Check sheet for the modelled part. Datum: model origin and axes. Units: mm. A direction names the side the tool comes from. Coordinates: 2 decimals unless noted, no trailing zeros. Write each loop counter-clockwise with the first axis right and the second up, starting at its lowest first coordinate (ties: lowest second). Pieces come first, ordered by that corner, then holes. Notation, with made-up numbers: (31, -19) -> (83, -19) arc R25 cw to (83, 5) -> close; hole circle Ø6 at (9, -40). An arc over 180 degrees is marked (long way). Put each result on its own line as item: value.
Autodesk Inventor part; units mm, degrees
ref_plane "YZ Plane" through (0, 0, 0) normal (1, 0, 0) x (0, 1, 0)
ref_plane "XZ Plane" through (0, 0, 0) normal (0, 1, 0) x (-1, 0, 0)
ref_plane "XY Plane" through (0, 0, 0) normal (0, 0, 1) x (1, 0, 0)
sketch "スケッチ1" plane through (0, 0, 0) normal (0, 1, 0) x (-1, 0, 0)
  line L0 (0, 0) -> (115, 0)
  line L1 (115, 0) -> (115, -157)
  line L2 (115, -157) -> (0, -157)
  line L3 (0, -157) -> (0, 0)
  line L4 (120, -162) -> (120, 5)
  line L5 (120, 5) -> (-5, 5)
  line L6 (-5, 5) -> (-5, -162)
  line L7 (-5, -162) -> (120, -162)
  dimension "d0" = 115
  dimension "d1" = 157
  dimension "d2" = 5
extrude "押し出し1" add sketch "スケッチ1" along normal blind 5 contours L0 L1 L2 L3 | L7 L6 L5 L4
sketch "スケッチ2" plane through (0, 5, 0) normal (0, 1, 0) x (1, 0, 0)
  line L0 (-120, -5) -> (5, -5)
  line L1 (5, -5) -> (5, 162)
  line L2 (5, 162) -> (-120, 162)
  line L3 (-120, 162) -> (-120, -5)
  line L4 (-115, 0) -> (0, 0)
  line L5 (0, 0) -> (0, 157)
  line L6 (0, 157) -> (-115, 157)
  line L7 (-115, 157) -> (-115, 0)
  line L8 (-115, 0) -> (-120, 0)
  line L9 (-120, 162) -> (-120, -5)
  line L10 (-115, 157) -> (-120, 157)
  point P0 (0, 0)
  dimension "d5" = 5
extrude "押し出し2" add sketch "スケッチ2" along normal blind 20 contours L3 L8 L4 L5 L6 L10 L2 L1 L0
sketch "スケッチ3" plane through (0, 5, -157) normal (-1, 0, 0) x (0, 0, 1)
  line L0 (0, 0) -> (0, 20)
  line L1 (0, 20) -> (3, 20)
  line L2 (0, 20) -> (157, 20)
  line L3 (3, 20) -> (3, 18.5)
  line L4 (3, 18.5) -> (0, 17)
  line L5 (78.5, 20) -> (78.5, -5)
  line L6 (-5, -5) -> (162, -5)
  line L7 (157, 20) -> (154, 20)
  line L8 (154, 20) -> (154, 18.5)
  line L9 (154, 18.5) -> (157, 17)
  line L10 (157, 0) -> (0, 0)
  line L11 (157, 0) -> (157, 20)
  line L12 (0, 20) -> (157, 20)
  line L13 (0, 0) -> (0, 20)
  point P0 (157, -5)
  point P1 (157, 17)
  point P2 (154, 20)
  dimension "d8" = 3
  dimension "d9" = 1.5
  dimension "d10" = 1.5
extrude "押し出し3" add sketch "スケッチ3" along normal blind 85 contours L0 L1 L3 L4 | L2 L11 L9 L8
sketch "スケッチ4" plane through (-120, 0, 5) normal (0, 0, 1) x (1, 0, 0)
  line L0 (120, 25) -> (35, 25)
  line L1 (65, 25) -> (25, 25)
  line L2 (25, 25) -> (25, 5)
  line L3 (25, 5) -> (65, 5)
  line L4 (65, 5) -> (65, 25)
  line L5 (0, 0) -> (0, 25)
  line L6 (0, 5) -> (120, 5)
  line L7 (25, 23) -> (65, 23)
  point P0 (120, 0)
  dimension "d13" = 65
  dimension "d14" = 40
  dimension "d15" = 0
  dimension "d16" = 2
extrude "押し出し4" cut sketch "スケッチ4" against normal blind 10 contours L4 L3 L2 L7
sketch "スケッチ5" plane through (0, 0, 0) normal (0, -1, 0) x (1, 0, 0)
  line L0 (-95, -116) -> (-55, -116)
  line L1 (-55, -116) -> (-55, -41)
  line L2 (-55, -41) -> (-95, -41)
  line L3 (-95, -41) -> (-95, -116)
  line L4 (-120, -162) -> (-120, 5)
  point P0 (0, 0)
  point P1 (-120, -78.5)
  point P2 (-95, -78.5)
  dimension "d19" = 65
  dimension "d20" = 75
  dimension "d21" = 25
  dimension "d22" = 0
extrude "押し出し5" cut sketch "スケッチ5" against normal through all
sketch "スケッチ6" plane through (5, 0, 5) normal (1, 0, 0) x (0, 0, -1)
  line L0 (5, 5) -> (5, 22)
  line L1 (5, 5) -> (30, 5)
  line L2 (30, 5) -> (30, 22)
  line L3 (30, 22) -> (5, 22)
  line L4 (5, 22) -> (5, 5)
  point P0 (5, 0)
  dimension "d25" = 25
  dimension "d26" = 0
extrude "押し出し6" cut sketch "スケッチ6" against normal up to surface (5 mm away)
sketch "スケッチ7" plane through (0, 0, 0) normal (0, -1, 0) x (1, 0, 0)
  circle A0 centre (-115, 15) radius 1.7
  circle A1 centre (0, 15) radius 1.7
  circle A2 centre (-115, -172) radius 1.7
  circle A3 centre (0, -172) radius 1.7
  line L0 (5, -162) -> (-120, -162)
  line L1 (-5, -162) -> (5, -162)
  line L2 (5, -162) -> (5, -177)
  line L3 (5, -177) -> (-5, -177)
  line L4 (-5, -177) -> (-5, -162)
  line L5 (-110, -162) -> (-120, -162)
  line L6 (-120, -162) -> (-120, -177)
  line L7 (-120, -177) -> (-110, -177)
  line L8 (-110, -177) -> (-110, -162)
  line L9 (-120, 5) -> (5, 5)
  line L10 (-120, 5) -> (-110, 5)
  line L11 (-110, 5) -> (-110, 20)
  line L12 (-110, 20) -> (-120, 20)
  line L13 (-120, 20) -> (-120, 5)
  line L14 (-5, 5) -> (5, 5)
  line L15 (5, 5) -> (5, 20)
  line L16 (5, 20) -> (-5, 20)
  line L17 (-5, 20) -> (-5, 5)
  line L18 (5, 5) -> (5, -162)
  line L19 (-120, -162) -> (-120, 5)
  circle A4 centre (120, -172) radius 1.7
  circle A5 centre (62.9804, -172) radius 1.525
  point P0 (0, 0)
  dimension "d29" = 3.4
  dimension "d30" = 3.4
  dimension "d31" = 3.4
  dimension "d32" = 3.4
  dimension "d33" = 5
  dimension "d34" = 5
  dimension "d35" = 5
  dimension "d36" = 5
  dimension "d37" = 5
  dimension "d38" = 5
  dimension "d39" = 5
  dimension "d40" = 5
  dimension "d41" = 5
  dimension "d42" = 5
  dimension "d43" = 5
  dimension "d44" = 5
  dimension "d45" = 10
  dimension "d46" = 10
  dimension "d47" = 10
  dimension "d48" = 10
  dimension "d56" = 0
  dimension "d57" = 0
  dimension "d60" = 57.0196
  dimension "d63" = 0
  dimension "d64" = 0
extrude "押し出し7" add sketch "スケッチ7" against normal blind 5 contours L2 L3 L4 L0 | L9 L17 L16 L15 | L8 L7 L6 L0 | L9 L13 L12 L11
fillet "フィレット1" radius 2 8 edges at (-110, 2.5, 5) (-5, 2.5, 5) (-110, 2.5, -162) (-5, 2.5, -162) (0, 5, -162) (-115, 5, -162) (-115, 5, 5) (0, 5, 5)
fillet "フィレット2" radius 1 37 edges at (5, 5, 13.5) (5, 16, 5) (5, 2.5, 20) (-57.5, 25, 5) (-110, 2.5, 20) (-120, 2.5, 20) (-5, 2.5, -177) (-57.5, 25, -162) (5, 25, -78.5) (5, 5, -170.5) (5, 16, -162) (-5.5858, 5.5858, -162.5858) (-5, 5, -170.5) (0, 5, -177) (-115, 5, -177) (-109.4142, 5.5858, -162.5858) (-110, 5, -170.5) (-120, 2.5, -177) (-110, 2.5, -177) (-120, 16, -162) (-120, 5, -170.5) (-120, 5, 13.5) (-120, 16, 5) (-109.4142, 5.5858, 5.5858) (-110, 5, 13.5) (-115, 5, 20) (-42.5, 25, -3) (-102.5, 25, 0) (0, 25, -78.5) (-42.5, 25, -154) (-102.5, 25, -157) (-85, 25, -155.5) (-85, 25, -1.5) (-95, 2.5, -41) (-55, 2.5, -41) (-55, 2.5, -116) (-95, 2.5, -116)
properties part number "pccase"
Q1. Depth check by flat-ended pin: P1, Ø3, axis at x = -87.5, z = -141, coming from the -Y side; P2, Ø6.5, axis at x = -2, z = -171, coming from the +Y side; P3, Ø0.6, axis at x = -23, y = 24, coming from the +Z side; P4, Ø4, axis at x = -72.5, y = 19.5, coming from the +Z side. Enter the tip coordinate at first touch or a pass-through.
Recorded:
P1: stops at y = 0
P2: stops at y = 5
P3: stops at z = 5
P4: stops at z = -157
Q2. Material ranges on line 1 along Z through (x, y) = (-115, 3.8); line 2 along Z through (x, y) = (-58, 4.5); line 3 along X through (y, z) = (1.5, -172), recorded low to high.
Recorded:
line 1: z = -177 to -173.7, -170.3 to 13.3, 16.7 to 20
line 2: z = -162 to -116, -41 to 5
line 3: x = -120 to -116.7, -113.3 to -110, -5 to -1.7, 1.7 to 5
Q3. Cross-section at A-A (x = -88.5). Record the cut outline in (y, z), plus the area to 3 significant figures.
Recorded:
outline: (0, -162) -> (24, -162) arc R1 ccw to (25, -161) -> (25, -158) arc R1 ccw to (24, -157) -> (5, -157) -> (5, -116) -> (0, -116) -> close; (0, -41) -> (5, -41) -> (5, 5) -> (0, 5) -> close; (23, 0) -> (24, 0) arc R1 ccw to (25, 1) -> (25, 4) arc R1 ccw to (24, 5) -> (23, 5) -> close
area: 569 mm2
Q4. Tool access check on faces 4 (the flat face through (-75, 2, -116)), 5 (the flat face through (-5, 2, 14)), 6 (the flat face through (-5, 2, -170)), 7 (the flat face through (-59, 14, -157)). Record the directions out of +Z, -Z, +X, -X, +Y, -Y that give a thin tool (end or side, any length) a straight path to the whole face; none if there is none.
Recorded:
face 4: +Y, -Y
face 5: +Z, +Y, -Y
face 6: -Z, +Y, -Y
face 7: -X
Q5. Cross-section at C-C (y = 19.5). Record the cut outline in (x, z).
Recorded:
outline: (-120, -161) arc R1 ccw to (-119, -162) -> (4, -162) arc R1 ccw to (5, -161) -> (5, -25) -> (0, -25) -> (0, -157) -> (-120, -157) -> close; (-120, 0) -> (-95, 0) -> (-95, 5) -> (-119, 5) arc R1 ccw to (-120, 4) -> close; (-55, 0) -> (5, 0) -> (5, 4) arc R1 ccw to (4, 5) -> (-55, 5) -> close
Q6. Mould release check, pull along Z, two halves, no side actions. Record for faces 1 (the flat face through (1, 2, -177)), 2 (the flat face through (-95, 2, -78)), 3 (the flat face through (-45, 12, 5)): released by +Z, released by -Z, zero draft, split by the parting line, or undercut.
Recorded:
face 1: released by -Z
face 2: undercut
face 3: released by +Z
Q7. Cross-section at D-D (x = -19). Record the cut outline in (y, z), plus the area to 3 significant figures.
Recorded:
outline: (0, -162) -> (24, -162) arc R1 ccw to (25, -161) -> (25, -155) arc R1 ccw to (24, -154) -> (23.5, -154) -> (22, -157) -> (5, -157) -> (5, 0) -> (22, 0) -> (23.5, -3) -> (24, -3) arc R1 ccw to (25, -2) -> (25, 4) arc R1 ccw to (24, 5) -> (0, 5) -> close
area: 1,050 mm2
Q8. Cross-section at B-B (z = -46). Record the cut outline in (x, y), plus the area to 3 significant figures.
Recorded:
outline: (-120, 0) -> (-95, 0) -> (-95, 5) -> (-120, 5) -> close; (-55, 0) -> (5, 0) -> (5, 24) arc R1 ccw to (4, 25) -> (1, 25) arc R1 ccw to (0, 24) -> (0, 5) -> (-55, 5) -> close
area: 525 mm2
